Read the model definition and answer for the solid it produces. Units are mm, in the model's axes. Face numbers are marked on the shaded views. Coordinates: 2 decimals unless noted, no trailing zeros. Order: outer loops, then holes, each group sorted by start corner. A loop starts at its lowest first (then second) coordinate and runs counter-clockwise, first axis right, second up. Notation, with made-up numbers: M 83,-37.75 L 125,-37.75 A17 cw 125,-18.75 Z; hole C 86,53 d1. An arc over 180 degrees is marked long. One line per question, with ' | ' between items. Start each with the question number.
1) The mould has two halves that part along Z. Classify the marked faces 1, 2, 3 and 4: +Z half, -Z half, draft (parallel to the pull), parting line (faces both ways), or undercut.
2) Find section D-D, the plane x = -13.75. Write down the section's boundary in (y, z) (1 decimal).
3) Given P1, Ø2.5, axis at y = 50.5, z = 23, coming from the -X side; P2, Ø5, axis at x = -5.5, z = 19.5, coming from the -Y side; P3, Ø1.4, axis at x = -11, y = 32.5, coming from the -Z side; P4, Ø5.5, axis at y = 71.12, z = 52.07, coming from the +X side, each flat-ended and moving along its own axis, determine where each tip first touches the part or whether it passes through.
4) Find section A-A, the plane x = -6.75. Write down the section's boundary in (y, z).
5) Consider probe 1 along X at (y, z) = (38, 5.5) (3 decimals); probe 2 along Z at (x, y) = (-12.1, 50.8); probe 3 along Y at (x, z) = (-11.5, 53.5). Determine where each line is inside the solid, lowest interval first.
6) Find section C-C, the plane y = 50.8. Write down the section's boundary in (x, z) (3 decimals).
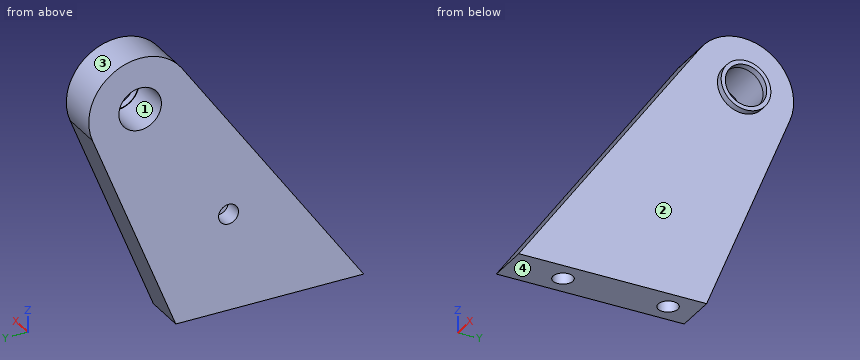
from build123d import *

# Parameters (mm, degrees)
SKETCH024_R     = 4.8895
PAD013_DEPTH    = 9.525
SKETCH034_R     = 5.715
SKETCH034_R_2   = 4.7625
PAD018_DEPTH    = 1.587
SKETCH035_R     = 2.286
POCKET013_DEPTH = 4.318
SKETCH073_R     = 2.286
POCKET035_DEPTH = 4.318


with BuildPart() as obj1:
    # Sketch024 → Pad013 (new body)
    with BuildSketch(Plane.YZ.offset(19.05)):
        with BuildLine():
            Line((12.125906, 0), (53.8632737741, 58.8988526596))
            ThreePointArc((74.4593338965, 47.6662832125), (69.1550841602, 62.43917278), (53.8632737741, 58.8988526596))
            Line((74.4593338965, 47.6662832125), (55.305906, 0))
            Line((55.305906, 0), (12.125906, 0))
        make_face()
        with Locations((63.5, 52.07)):
            Circle(SKETCH024_R, mode=Mode.SUBTRACT)
    extrude(amount=PAD013_DEPTH)

    # Sketch034 (on Face6 of Pad013) → Pad018 (join)
    with BuildSketch(Plane(origin=(19.05, 0, 0), x_dir=(0, 1, 0), z_dir=(-1, 0, 0))):
        with Locations((63.5, -52.07)):
            Circle(SKETCH034_R)
        with Locations((63.5, -52.07)):
            Circle(SKETCH034_R_2, mode=Mode.SUBTRACT)
    extrude(amount=PAD018_DEPTH)

    # Sketch035 (on Face3 of Pad018) → Pocket013 (cut)
    with BuildSketch(Plane.YX):
        with Locations((24.85996, 23.8125)):
            Circle(SKETCH035_R)
        with Locations((49.014852994, 23.8125)):
            Circle(SKETCH035_R)
    extrude(amount=-POCKET013_DEPTH, mode=Mode.SUBTRACT)

    # Sketch073 → Pocket035 (cut)
    with BuildSketch(Plane.YZ.offset(28.575)):
        with Locations((43.18, 22.225)):
            Circle(SKETCH073_R)
    extrude(amount=-POCKET035_DEPTH, mode=Mode.SUBTRACT)


with BuildPart() as obj1_1:
    # Body005 placement: moved
    add(obj1.part.moved(Location((-4.57, 7.62, 0))))


with BuildPart() as obj2:
    # Part__Mirroring: instance of obj1
    add(obj1_1.part.mirror(Plane(origin=(0, 0, 0), x_dir=(0, -1, 0), z_dir=(1, 0, 0))))


with BuildPart() as obj2_1:
    # Part__Mirroring placement: moved
    add(obj2.part.moved(Location((9.4, 0, 0))))


solid = obj2_1.part
Report:
1) face 1: undercut | face 2: draft | face 3: parting line | face 4: -Z half
2) outline: M 19.7,0 L 62.9,0 L 82.1,47.7 A11.8 ccw 61.5,58.9 Z; hole C 50.8,22.2 d4.6; hole C 71.1,52.1 d9.8
3) P1: stops at x = -10.29 | P2: stops at y = 31.79 | P3: stops at z = 4.32 | P4: passes through
4) outline: M 19.75,0 L 62.93,0 L 82.08,47.67 A11.81 ccw 61.48,58.9 Z; hole C 71.12,52.07 d9.78
5) probe 1: x = -14.605 to -5.08 | probe 2: z = 0 to 19.94, 24.51 to 43.82 | probe 3: y = 57.66 to 66.44, 75.8 to 82.84
6) outline: M -14.605,0 L -5.08,0 L -5.08,43.823 L -14.605,43.823 L -14.605,24.511 L -10.287,24.511 L -10.287,19.939 L -14.605,19.939 Z
